Build history of the part. All positions in model axes, mm. Round coordinates to 2 decimals unless told otherwise and drop trailing zeros. Write each loop counter-clockwise with the first axis right and the second up, starting at its lowest first coordinate (ties: lowest second). Pieces come first, ordered by that corner, then holes. Notation, with made-up numbers: (-33, 10) -> (-18, 10) arc R31 ccw to (-18, 45) -> close; hole circle Ø1 at (73.5, -19.5). An arc over 180 degrees is marked (long way). Return JSON: item names as keys, results as strings.
from build123d import *

# Parameters (mm, degrees)
SKETCH1_R               = 50.8
BOSS_EXTRUDE1_DEPTH     = 50.8
SKETCH2_W               = 101.6
SKETCH2_H               = 50.8
SKETCH2_R               = 16.256
CUT_EXTRUDE1_DEPTH      = 51.8
CUT_EXTRUDE1_DEPTH_BACK = 51.8
SKETCH3_R               = 16.256
CUT_EXTRUDE2_DEPTH      = 50.8


with BuildPart() as part:
    # Sketch1 → Boss-Extrude1 (new body)
    with BuildSketch(Plane(origin=(0, 0, 0), x_dir=(1, 0, 0), z_dir=(0, 1, 0))):
        Circle(SKETCH1_R)
    extrude(amount=BOSS_EXTRUDE1_DEPTH)

    # Sketch2 → Cut-Extrude1 (cut, two sides)
    with BuildSketch(Plane.XY) as cut_extrude1_sk:
        with Locations((0, 25.4)):
            Rectangle(SKETCH2_W, SKETCH2_H)
        with Locations((0, 25.4)):
            Circle(SKETCH2_R, mode=Mode.SUBTRACT)
    extrude(amount=CUT_EXTRUDE1_DEPTH, mode=Mode.SUBTRACT)
    extrude(cut_extrude1_sk.sketch, amount=-CUT_EXTRUDE1_DEPTH_BACK, mode=Mode.SUBTRACT)

    # Sketch3 → Cut-Extrude2 (cut)
    with BuildSketch(Plane.XY):
        with Locations((0, 25.4)):
            Circle(SKETCH3_R)
    extrude(amount=-CUT_EXTRUDE2_DEPTH, mode=Mode.SUBTRACT)


solid = part.part
Q1. Pin check, flat tips, straight feed: pin 1 Ø12 at (x, z) = (-9, 33) entering from -Y; pin 2 Ø2 at (y, z) = (37, 28) entering from +X; pin 3 Ø2 at (y, z) = (17.5, 14) entering from +X; pin 4 Ø4 at (x, y) = (-11.5, 32) entering from -Z. Stop position of each tip, or through.
Verdict:
{"pin 1": "stops at y = 9.42", "pin 2": "stops at x = 12.32", "pin 3": "stops at x = 14.72", "pin 4": "stops at z = 0"}
Q2. Wall check: L1, parallel to Z at x = -1, y = 20.5; L2, parallel to Z at x = -4, y = 26; L3, parallel to X at y = 23, z = 32. Give the ranges that are in metal, low to high.
Verdict:
{"L1": "z = 0 to 50.79", "L2": "z = 0 to 50.64", "L3": "x = -16.08 to 16.08"}
Q3. Saw through at B-B on y = 25.4. List the corners of the cut face in (x, z), then the cut area to 3 significant figures.
Verdict:
{"outline": "(-16.26, 0) -> (16.26, 0) -> (16.26, 48.13) arc R50.8 ccw to (-16.26, 48.13) -> close", "area": "1,620 mm²"}
Q4. Saw through at A-A on z = 43. List the corners of the cut face in (x, y).
Verdict:
{"outline": "circle Ø32.51 at (0, 25.4)"}
Q5. Saw through at C-C on x = -11. List the corners of the cut face in (y, z).
Verdict:
{"outline": "(13.43, 0) -> (37.37, 0) -> (37.37, 49.59) -> (13.43, 49.59) -> close"}
